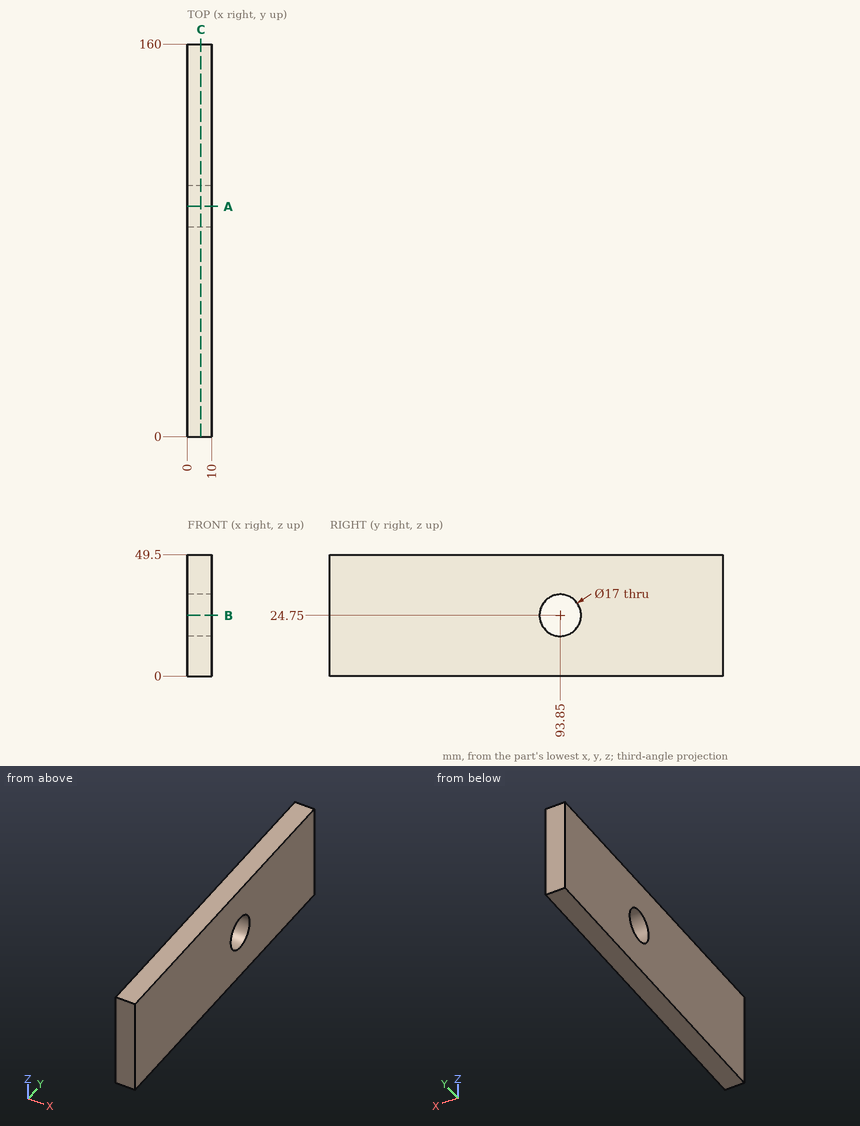
Answer from the drawing. Dimensions are ordinates in mm from the lowest x, y and z of the part. Give positions to 0.01 mm unless a question says otherwise; leave off trailing zeros. Order: outer loops, then holes, each group sorted by start corner. A loop starts at its lowest first (then second) coordinate and runs counter-clockwise, first axis right, second up. Notation, with made-up numbers: (13, 18) -> (34, 18) arc R29 cw to (34, 39) -> close; hole circle Ø9 at (5.5, 75.25). An arc over 180 degrees is marked (long way). Answer as a JSON object with one key per item and string values. Group by question number.
1. A flat-ended cylindrical pin translates along its axis: pin 1 Ø1.5 at (y, z) = (133.5, 18.5) entering from -X. Find the tip coordinate at first contact, or state that the pin passes through.
2. Section B-B on z = 24.75 is taken. Determine the outline of the cut face in (x, y), plus the area to 3 significant figures.
3. Consider line 1 along Z through (x, y) = (5.5, 93.85); line 2 along Y through (x, z) = (1.75, 23); line 3 along Z through (x, y) = (5.5, 89). Determine where each line is inside the solid, lowest interval first. Write a range as [from, to].
4. Section C-C on x = 5.5 is taken. Determine the outline of the cut face in (y, z), plus the area to 3 significant figures.
5. Section A-A on y = 93.85 is taken. Determine the outline of the cut face in (x, z), plus the area to 3 significant figures.
Result sheet:
{
 "1": {"pin 1": "stops at x = 0"},
 "2": {"outline": "(0, 0) -> (10, 0) -> (10, 85.35) -> (0, 85.35) -> close; (0, 102.35) -> (10, 102.35) -> (10, 160) -> (0, 160) -> close", "area": "1,430 mm^2"},
 "3": {"line 1": "z = [0, 16.25], [33.25, 49.5]", "line 2": "y = [0, 85.53], [102.17, 160]", "line 3": "z = [0, 17.77], [31.73, 49.5]"},
 "4": {"outline": "(0, 0) -> (160, 0) -> (160, 49.5) -> (0, 49.5) -> close; hole circle Ø17 at (93.85, 24.75)", "area": "7,690 mm^2"},
 "5": {"outline": "(0, 0) -> (10, 0) -> (10, 16.25) -> (0, 16.25) -> close; (0, 33.25) -> (10, 33.25) -> (10, 49.5) -> (0, 49.5) -> close", "area": "325 mm^2"}
}
